Can you work these out from the model? Positions are in its coordinate system, mm. A direction names the side the tool comes from. Coordinates: 2 decimals unless noted, no trailing zeros. Order: outer loops, then holes, each group sorted by start corner. A loop starts at its lowest first (then second) coordinate and runs counter-clockwise, first axis right, second up. Notation, with made-up numbers: M -27.75,38 L -16.75,38 A8 ccw -16.75,42 Z; hole C 75.5,22.25 d4. An arc over 180 degrees is marked long. Answer as a JSON object with one key per item and string values.
from build123d import *

# Parameters (mm, degrees)
SKETCH2_R            = 3.75
CUT_EXTRUDE1_DEPTH   = 6
CUT_EXTRUDE2_START   = 7.858117
SKETCH3_R            = 1.5
CUT_EXTRUDE2_DEPTH   = 8.141883
FILLET1_R            = 3
FILLET3_R            = 2.5
FILLET1_OF_MIRROR1_R = 3
FILLET3_OF_MIRROR1_R = 2.5


with BuildPart() as part:
    # Sketch1 → Revolve1 (revolve)
    with BuildSketch(Plane(origin=(0, 0, 0), x_dir=(0, 0, -1), z_dir=(1, 0, 0))):
        Polygon((0, 8), (0, 40), (-20, 40), (-20, 37), (-5, 35), (-5, 16), (-19.5, 16), (-19.5, 8), align=None)
    revolve1 = revolve(axis=Axis((0, 0, 30), (0, 0, -1)))

    # Sketch2 → Cut-Extrude1 (cut, through all)
    with BuildSketch(Plane.XY.offset(5)):
        with Locations((0, 25)):
            Circle(SKETCH2_R)
        with Locations((17.67766953, 17.67766953)):
            Circle(SKETCH2_R)
        with Locations((25, 0)):
            Circle(SKETCH2_R)
        with Locations((17.67766953, -17.67766953)):
            Circle(SKETCH2_R)
        with Locations((0, -25)):
            Circle(SKETCH2_R)
        with Locations((-17.67766953, -17.67766953)):
            Circle(SKETCH2_R)
        with Locations((-25, 0)):
            Circle(SKETCH2_R)
        with Locations((-17.67766953, 17.67766953)):
            Circle(SKETCH2_R)
    cut_extrude1 = extrude(amount=-CUT_EXTRUDE1_DEPTH, mode=Mode.SUBTRACT)

    # Sketch3 → Cut-Extrude2 (cut)
    with BuildSketch(Plane(origin=(0, 0, 0), x_dir=(1, 0, 0), z_dir=(0, 1, 0)).offset(CUT_EXTRUDE2_START)):
        with Locations((0, -14)):
            Circle(SKETCH3_R)
    cut_extrude2 = extrude(amount=CUT_EXTRUDE2_DEPTH, mode=Mode.SUBTRACT)

    # Fillet1
    fillet1_edges = [part.edges().sort_by_distance(p)[0] for p in [
        (0, -35, 5),
    ]]
    fillet(fillet1_edges, radius=FILLET1_R)

    # Fillet3
    fillet3_edges = [part.edges().sort_by_distance(p)[0] for p in [
        (0, -16, 19.5),
    ]]
    fillet(fillet3_edges, radius=FILLET3_R)

    # Mirror1: Revolve1, Cut-Extrude1, Cut-Extrude2 across plane
    add(revolve1.mirror(Plane.XY))
    add(cut_extrude1.mirror(Plane.XY), mode=Mode.SUBTRACT)
    add(cut_extrude2.mirror(Plane.XY), mode=Mode.SUBTRACT)

    # Fillet1 of Mirror1
    fillet1_of_mirror1_edges = [part.edges().sort_by_distance(p)[0] for p in [
        (0, -35, -5),
    ]]
    fillet(fillet1_of_mirror1_edges, radius=FILLET1_OF_MIRROR1_R)

    # Fillet3 of Mirror1
    fillet3_of_mirror1_edges = [part.edges().sort_by_distance(p)[0] for p in [
        (0, -16, -19.5),
    ]]
    fillet(fillet3_of_mirror1_edges, radius=FILLET3_OF_MIRROR1_R)


solid = part.part
Item 1: If we mould it in two halves opening along X, with no side actions, what happens to faces 1 (the flat face through (-35.4, 11.7, -20)), 2 (the cylindrical face through (-18.491, 14.017, -0.07))? For each: pulls with the +X half, pulls with the -X half, needs draft (parallel to the pull), parting line crosses it, or undercut.
Answers follow:
{"face 1": "needs draft", "face 2": "undercut"}
Item 2: Please list where these lines run through material, in increasing order: line 1 (Z direction, x = 0, y = 12.25); line 2 (Y direction, x = 14.5, z = 2); line 3 (Y direction, x = 11, z = 14.5).
Answers follow:
{"line 1": "z = -19.5 to -15.5, -12.5 to 12.5, 15.5 to 19.5", "line 2": "y = -37.28 to -19.67, -15.69 to 15.69, 19.67 to 37.28", "line 3": "y = -38.46 to -34.56, -11.62 to 11.62, 34.56 to 38.46"}
Item 3: I want a section at A-A, the plane z = 14. Write out the boundary of the cut face in (x, y).
Answers follow:
{"outline": "C 0,0 d80; M -1.5,7.86 L -1.5,15.93 A16 ccw long 1.5,15.93 L 1.5,7.86 A8 cw long Z; hole C 0,0 d72.4"}
Item 4: Which directions (+Z, -Z, +X, -X, +Y, -Y) give clear straight access to the entire face, cutting with the end or side of a thin tool? Please do faces 3 (the flat face through (-7, -15, -5)), 4 (the flat face through (-6, 6, 19.5)), 5 (the cylindrical face through (-0.325, 11.872, -15.464)).
Answers follow:
{"face 3": "-Z", "face 4": "+Z", "face 5": "none"}
Item 5: I want a section at B-B, the plane x = 0. Give the number of separate pieces and of enclosed holes in the cut face, plus the area to 3 significant figures.
Answers follow:
{"separate pieces": "6", "enclosed holes": "0", "area": "1,150 mm^2"}
Item 6: I'm going to push flat-ended pins straight in: pin 1 (8 mm diameter, centred on y = 30.5, z = 9, fed in from -X); pin 2 (19.5 mm diameter, centred on x = 8, y = -12.5, fed in from +Z); pin 3 (8 mm diameter, centred on x = 1, y = -2, fed in from +Z); pin 4 (5 mm diameter, centred on x = -16, z = 1, fed in from +Y). Where does each tip first touch, or does it pass through?
Answers follow:
{"pin 1": "stops at x = -29.96", "pin 2": "stops at z = 19.5", "pin 3": "passes through", "pin 4": "stops at y = 37.65"}
